Autodesk Inventor part; units mm, degrees
ref_plane "YZ Plane" through (0, 0, 0) normal (1, 0, 0) x (0, 1, 0)
ref_plane "XZ Plane" through (0, 0, 0) normal (0, 1, 0) x (-1, 0, 0)
ref_plane "XY Plane" through (0, 0, 0) normal (0, 0, 1) x (1, 0, 0)
sketch "Sketch1" plane through (0, 0, 0) normal (0, 1, 0) x (-1, 0, 0)
  line L0 (-15, 22.5) -> (15, 22.5)
  line L1 (15, 22.5) -> (15, -22.5)
  line L2 (15, -22.5) -> (-15, -22.5)
  line L3 (-15, -22.5) -> (-15, 22.5)
  line L4 (-15, 22.5) -> (15, -22.5) construction
  line L5 (15, 22.5) -> (-15, -22.5) construction
  circle A0 centre (15, 22.5) radius 3.5
  circle A1 centre (-15, 22.5) radius 3.5
  circle A2 centre (15, -22.5) radius 3.5
  circle A3 centre (-15, -22.5) radius 3.5
  line L6 (22.5, 30) -> (-22.5, 30)
  line L7 (-22.5, 30) -> (-22.5, -30)
  line L8 (-22.5, -30) -> (22.5, -30)
  line L9 (22.5, -30) -> (22.5, 30)
  line L10 (22.5, 30) -> (-22.5, -30) construction
  line L11 (-22.5, 30) -> (22.5, -30) construction
  circle A4 centre (15, 22.5) radius 1.45
  circle A5 centre (15, -22.5) radius 1.45
  circle A6 centre (-15, 22.5) radius 1.45
  circle A7 centre (-15, -22.5) radius 1.45
  point P0 (0, 0)
  point P1 (-11.5, 22.5)
  point P2 (-15, 19)
  point P3 (-15, -19)
  point P4 (-11.5, -22.5)
  point P5 (11.5, -22.5)
  point P6 (15, -19)
  point P7 (15, 19)
  point P8 (11.5, 22.5)
  dimension "d0" = 45
  dimension "d1" = 30
  dimension "d2" = 7
  dimension "d3" = 7
  dimension "d4" = 7
  dimension "d5" = 7
  dimension "d6" = 7.5
  dimension "d7" = 7.5
  dimension "d8" = 2.9
  dimension "d9" = 2.9
  dimension "d10" = 2.9
  dimension "d11" = 2.9
extrude "Extrusion1" add sketch "Sketch1" against normal blind 5 contours A6 L3 A1 L0 | L0 A1 L3 A6 | A0 L1 A4 L0 | L0 A4 L1 A0 | A3 L2 A7 L3 | L3 A7 L2 A3 | A2 L2 A5 L1 | L1 A5 L2 A2
extrude "Extrusion2" add sketch "Sketch1" along normal blind 4 contours A6 L3 A1 L0 | L0 A1 L3 A6 | L0 A0 L1 A2 L2 A3 L3 A1 | A0 L1 A4 L0 | L0 A4 L1 A0 | A3 L2 A7 L3 | L3 A7 L2 A3 | A2 L2 A5 L1 | L1 A5 L2 A2 | L9 L8 L7 L6
sketch "Sketch2" plane through (0, 4, 0) normal (0, 1, 0) x (1, 0, 0)
  line L0 (-10, -30) -> (-5, -30)
  line L1 (-5, -30) -> (-5, 30)
  line L2 (-5, 30) -> (-10, 30)
  line L3 (-10, 30) -> (-10, -30)
  line L4 (-10, -30) -> (-5, 30) construction
  line L5 (-5, -30) -> (-10, 30) construction
  point P0 (0, 0)
  point P1 (-7.5, 0)
  dimension "d39" = 60
  dimension "d40" = 5
  dimension "d41" = 5
extrude "Extrusion3" add sketch "Sketch2" along normal blind 100
sketch "Sketch3" plane through (-5, 4, 30) normal (1, 0, 0) x (0, 0, -1)
  line L0 (30, 100) -> (30, 82.5)
  line L1 (16.25, 68.75) -> (43.75, 68.75)
  line L2 (43.75, 68.75) -> (43.75, 96.25)
  line L3 (43.75, 96.25) -> (16.25, 96.25)
  line L4 (16.25, 96.25) -> (16.25, 68.75)
  line L5 (16.25, 68.75) -> (43.75, 96.25) construction
  line L6 (43.75, 68.75) -> (16.25, 96.25) construction
  circle A0 centre (16.25, 96.25) radius 1.25
  circle A1 centre (43.75, 96.25) radius 1.25
  circle A2 centre (16.25, 68.75) radius 1.25
  circle A3 centre (43.75, 68.75) radius 1.25
  circle A4 centre (30, 82.5) radius 13.5
  circle A5 centre (16.25, 96.25) radius 3
  circle A6 centre (43.75, 96.25) radius 3
  circle A7 centre (16.25, 68.75) radius 3
  circle A8 centre (43.75, 68.75) radius 3
  line L7 (0, 100) -> (60, 100)
  line L8 (60, 0) -> (60, 100)
  point P0 (30, -4)
  dimension "d19" = 27.5
  dimension "d20" = 27.5
  dimension "d21" = 2.5
  dimension "d22" = 2.5
  dimension "d23" = 2.5
  dimension "d24" = 2.5
  dimension "d26" = 27
  dimension "d27" = 6
  dimension "d28" = 6
  dimension "d29" = 6
  dimension "d30" = 6
  dimension "d42" = 17.5
  dimension "d53" = 30
extrude "Extrusion4" cut sketch "Sketch3" against normal blind 60 contours L4 A2 L1 | L1 A2 L4 | A3 L2 L1 | L1 L2 A3 | A0 L3 L4 | L4 L3 A0 | A1 L3 L2 | L2 L3 A1 | A4
extrude "Extrusion5" add sketch "Sketch3" along normal blind 5 contours A2 L4 A7 L1 | L1 A7 L4 A2 | A8 L2 A3 L1 | L1 A3 L2 A8 | A5 L3 A0 L4 | L4 A0 L3 A5 | A6 L3 A1 L2 | L2 A1 L3 A6
fillet "Fillet1" radius 10 2 edges at (-7.5, 104, -30) (-7.5, 104, 30)
sketch "Sketch6" plane through (-10, 4, 30) normal (0, 0, 1) x (-1, 0, 0)
  line L0 (-5, 0) -> (-5, -90)
  line L1 (-5, -60) -> (-20, 0)
  line L2 (12.5, 0) -> (-32.5, 0)
  line L3 (-5, -36) -> (-14, 0)
  line L4 (-32.5, 0) -> (12.5, 0)
  line L5 (12.5, 4) -> (-32.5, 4)
  point P0 (-10, 4)
  point P1 (-10, 0)
  dimension "d50" = 40
  dimension "d52" = 15
  dimension "d54" = 60
extrude "Extrusion7" add sketch "Sketch6" against normal up to surface (60 mm away) contours L0 L1 L2 L3
fillet "Fillet2" radius 10 4 edges at (22.5, 2, 30) (-22.5, 2, 30) (22.5, 2, -30) (-22.5, 2, -30)
properties part number "Camera_holder"
Source: CAD feature listing. Evaluate the final solid. Frame: model axes, mm. A direction names the side the tool comes from. Coordinates: 2 decimals unless noted, no trailing zeros. Write each loop counter-clockwise with the first axis right and the second up, starting at its lowest first coordinate (ties: lowest second). Pieces come first, ordered by that corner, then holes. Notation, with made-up numbers: (-24.75, 46) -> (13.25, 46) arc R22 cw to (13.25, 76) -> close; hole circle Ø5 at (31, -16). An arc over 180 degrees is marked (long way). Return JSON: item names as keys, results as strings. Group by question number.
1) Ray query, line 1 along Y through (x, z) = (-7.25, 13.75); line 2 along Z through (x, y) = (15, -1.25); line 3 along X through (y, z) = (-2.75, -22.5). Return the intervals inside material, ascending.
2) Mould query, pull axis X, two halves, no side actions, for faces 1 (the face through (13.661, -0.563, 23.055)), 2 (the face through (-3.6, 36.3, -30)), 3 (the face through (-5, 74.8, 7.1)). Classes: +X half, -X half, draft (parallel to the pull), parting line (faces both ways), or undercut.
3) Set-up query: faces 4 (the face through (-5, 22, 0)), 5 (the face through (-10, 53, 0)), 6 (the face through (-2.54, 103.18, -13.1)), 7 (the face through (13.12, -2.46, -19.55)). Return all of +Z, -Z, +X, -X, +Y, -Y with unobstructed straight access to the full face (end or side cutting, diameter ignored); none if empty.
4) Section query B-B, the plane z = 22.5. Return loops of the section in (x, y).
5) Section query C-C, the plane x = 15. Return loops of the section in (y, z), plus the area to 3 significant figures.
6) Contact query for flat-ended pins moving along their axis: P1, Ø3, axis at y = 73.5, z = -8, coming from the +X side; P2, Ø3.5, axis at x = -15, z = -22.5, coming from the +Y side; P3, Ø1.5, axis at y = 72.75, z = -13.75, coming from the -X side; P4, Ø11, axis at y = 29.5, z = -2, coming from the +X side. Output: stop coordinate, or through.
7) Section query A-A, the plane z = 0. Return loops of the section in (x, y).
8) Section query D-D, the plane y = 83. Return loops of the section in (x, z), plus the area to 3 significant figures.
From the geometry:
{
 "1": {"line 1": "0 to 71.5, 74 to 99, 101.5 to 104", "line 2": "-26 to -23.95, -21.05 to -19, 19 to 21.05, 23.95 to 26", "line 3": "-18.5 to -16.45, -13.55 to -11.5, 11.5 to 13.55, 16.45 to 18.5"},
 "2": {"face 1": "undercut", "face 2": "draft", "face 3": "+X half"},
 "3": {"face 4": "+Z, -Z", "face 5": "+Z, -Z, -X, +Y", "face 6": "+X", "face 7": "-Y"},
 "4": {"outline": "(-22.18, 0) -> (-18.5, 0) -> (-18.5, -5) -> (-16.45, -5) -> (-16.45, 4) -> (-22.18, 4) -> close; (-13.55, -5) -> (-11.5, -5) -> (-11.5, 0) -> (11.5, 0) -> (11.5, -5) -> (13.55, -5) -> (13.55, 4) -> (10, 4) -> (-5, 64) -> (-5, 103.68) -> (-10, 103.68) -> (-10, 4) -> (-13.55, 4) -> close; (16.45, -5) -> (18.5, -5) -> (18.5, 0) -> (22.18, 0) -> (22.18, 4) -> (16.45, 4) -> close; hole (-5, 4) -> (4, 4) -> (-5, 40) -> close"},
 "5": {"outline": "(-5, -26) -> (0, -26) -> (0, -29.68) -> (4, -29.68) -> (4, -23.95) -> (-5, -23.95) -> close; (-5, -21.05) -> (4, -21.05) -> (4, 21.05) -> (-5, 21.05) -> (-5, 19) -> (0, 19) -> (0, -19) -> (-5, -19) -> close; (-5, 23.95) -> (4, 23.95) -> (4, 29.68) -> (0, 29.68) -> (0, 26) -> (-5, 26) -> close", "area": "255 mm²"},
 "6": {"P1": "x = -5", "P2": "y = 4", "P3": "through", "P4": "x = 5"},
 "7": {"outline": "(-22.5, 0) -> (22.5, 0) -> (22.5, 4) -> (10, 4) -> (-5, 64) -> (-5, 73) -> (-10, 73) -> (-10, 4) -> (-22.5, 4) -> close; (-10, 100) -> (-5, 100) -> (-5, 104) -> (-10, 104) -> close; hole (-5, 4) -> (4, 4) -> (-5, 40) -> close"},
 "8": {"outline": "(-10, -30) -> (-5, -30) -> (-5, -13.04) -> (-10, -13.04) -> close; (-10, 13.04) -> (-5, 13.04) -> (-5, 30) -> (-10, 30) -> close", "area": "170 mm²"}
}
